Check sheet for the modelled part. Datum: model origin and axes. Units: mm. Face numbers are marked on the shaded views. A direction names the side the tool comes from. Give positions to 0.01 mm unless a question says otherwise; leave off trailing zeros. Order: outer loops, then holes, each group sorted by start corner. A loop starts at its lowest first (then second) coordinate and runs counter-clockwise, first axis right, second up. Notation, with made-up numbers: (-38, 65.25) -> (-18, 65.25) arc R19 ccw to (-18, 89.25) -> close; hole circle Ø9 at (36, 63.25). An arc over 180 degrees is marked (long way). Answer in a Markdown table with one row per item. Add a question column.
(1) Set-up check for the marked faces 1, 2 and 3: record each of +Z, -Z, +X, -X, +Y, -Y from which the full face is reachable in a straight line by a thin tool's end or side.
(2) Cross-section at B-B (z = -14.5). Record the cut outline in (x, y), then the cut area to 3 significant figures.
(3) Go/stop test with flat-tipped pins: pin 1 (1.2 mm diameter, centred on y = -0.5, z = -19.5, fed in from +X); pin 2 (4 mm diameter, centred on y = 3, z = -6, fed in from +X); pin 3 (6 mm diameter, centred on y = -1, z = -8, fed in from -X). Record where each tip stops, or that it passes through.
(4) Cross-section at A-A (x = 0). Record the cut outline in (y, z), then the cut area to 3 significant figures.
(5) Release check for a two-part mould opening along Z. For the marked faces 4, 5 and 6 record: released by +Z, released by -Z, zero draft, split by the parting line, or undercut.
(6) Cross-section at D-D (z = -19). Record the cut outline in (x, y), then the cut area to 3 significant figures.
(7) Thickness scan on L1, parallel to Z at x = 6.25, y = 2.75; L2, parallel to X at y = 0.25, z = -3.5; L3, parallel to Z at x = -2.5, y = 3.25. Record the ranges inside material, lowest first. Write a range as [from, to].
(8) Cross-section at C-C (z = -5). Record the cut outline in (x, y), then the cut area to 3 significant figures.
Autodesk Inventor part; units mm, degrees
ref_plane "TopPlane" through (0, 0, 1.75) normal (0, 0, 1) x (1, 0, 0)
ref_plane "YZ Plane" through (0, 0, 0) normal (1, 0, 0) x (0, 1, 0)
ref_plane "XZ Plane" through (0, 0, 0) normal (0, 1, 0) x (-1, 0, 0)
sketch "BaseBottom" plane through (0, 0, 0) normal (0, 0, 1) x (1, 0, 0)
  circle A0 centre (0, 0) radius 9
  dimension "d0" = 18
ref_plane "TopPlane" through (0, 0, 1.75) normal (0, 0, 1) x (1, 0, 0)
sketch "BaseTop" plane through (0, 0, 1.75) normal (0, 0, 1) x (1, 0, 0)
  circle A0 centre (0, 0) radius 7
  dimension "d4" = 14
loft "BaseFeature" add profiles "BaseBottom", "BaseTop"
sketch "Light" plane through (0, 0, 1.75) normal (0, 0, 1) x (1, 0, 0)
  circle A0 centre (0, 0) radius 9
  circle A1 centre (0, 0) radius 6
  dimension "d9" = 12
extrude "LightFeature" add sketch "Light" along normal blind 0.1 contours A1
sketch "Thread" plane through (0, 0, 0) normal (0, 0, -1) x (-1, 0, 0)
  circle A0 centre (0, 0) radius 8
  dimension "d12" = 16
extrude "ThreadFeature" add sketch "Thread" along normal blind 12
sketch "Body" plane through (0, 0, -12) normal (0, 0, -1) x (-1, 0, 0)
  circle A0 centre (0, 0) radius 7.5
  dimension "d15" = 15
extrude "BodyFeature" add sketch "Body" along normal blind 3
sketch "TerminalsBase" plane through (0, 0, -15) normal (0, 0, -1) x (-1, 0, 0)
  circle A0 centre (0, 0) radius 6
  dimension "d18" = 12
extrude "TerminalsBaseFeature" add sketch "TerminalsBase" along normal blind 2.25
sketch "Terminals" plane through (0, 0, -17.25) normal (0, 0, -1) x (-1, 0, 0)
  line L0 (-6, -2) -> (6, -2)
  line L1 (6, -2) -> (6, 2)
  line L2 (6, 2) -> (-6, 2)
  line L3 (-6, 2) -> (-6, -2)
  line L4 (-6, -2) -> (6, 2) construction
  line L5 (6, -2) -> (-6, 2) construction
  circle A0 centre (0, 0) radius 6
  dimension "d21" = 4
extrude "TerminalsFeature" add sketch "Terminals" along normal blind 4 contours L3 A0 L0 | A0 L2 L0 | L3 L2 A0 | A0 L1 L0 | A0 L2 L1
properties part number "PilotLight"
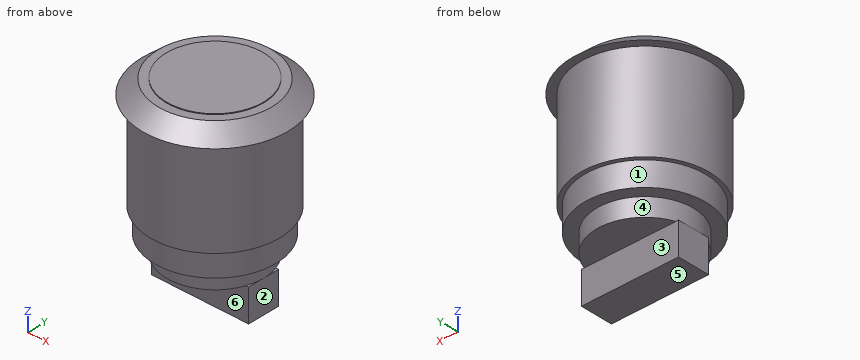
Answer below:
| question | item | result |
|---|---|---|
| 1 | face 1 | -Z |
| 1 | face 2 | -Z, +X, +Y, -Y |
| 1 | face 3 | -Z, +X, -X, +Y |
| 2 | outline | circle Ø15 at (0, 0) |
| 2 | area | 177 mm² |
| 3 | pin 1 | stops at x = 6 |
| 3 | pin 2 | stops at x = 7.94 |
| 3 | pin 3 | stops at x = -8 |
| 4 | outline | (-9, 0) -> (-8, 0) -> (-8, -12) -> (-7.5, -12) -> (-7.5, -15) -> (-6, -15) -> (-6, -17.25) -> (-2, -17.25) -> (-2, -21.25) -> (2, -21.25) -> (2, -17.25) -> (6, -17.25) -> (6, -15) -> (7.5, -15) -> (7.5, -12) -> (8, -12) -> (8, 0) -> (9, 0) -> (7, 1.75) -> (6, 1.75) -> (6, 1.85) -> (-6, 1.85) -> (-6, 1.75) -> (-7, 1.75) -> close |
| 4 | area | 309 mm² |
| 5 | face 4 | undercut |
| 5 | face 5 | released by -Z |
| 5 | face 6 | zero draft |
| 6 | outline | (-6, -2) -> (6, -2) -> (6, 2) -> (-6, 2) -> close |
| 6 | area | 48.0 mm² |
| 7 | L1 | z = [-15, 1.75] |
| 7 | L2 | x = [-8, 8] |
| 7 | L3 | z = [-17.25, 1.85] |
| 8 | outline | circle Ø16 at (0, 0) |
| 8 | area | 201 mm² |
